The listing builds one solid part. Answer for the finished solid, in the listing's coordinates (mm). A direction names the side the tool comes from. Give positions to 0.01 mm unless a question says otherwise; leave off trailing zeros. Order: outer loops, then holes, each group sorted by start corner. A loop starts at its lowest first (then second) coordinate and runs counter-clockwise, first axis right, second up. Notation, with made-up numbers: (37, 80) - (63, 80) arc R28 cw to (63, 112) - close; hole circle Ø8 at (51, 19.5). An arc over 180 degrees is marked (long way). Use a Markdown table: item, result. Add a question column.
1) The mould has two halves that part along Z. Classify faces 6 (the face through (4.8, 22, -98)), 7 (the face through (4, 33, 0)), 8 (the face through (28.946, 30.8, -86.999)): released by +Z, released by -Z, zero draft, split by the parting line, or undercut.
2) Find section A-A, the plane y = 41. Determine the outline of the cut face in (x, z).
3) Straight lines are drawn through the part: line 1 (X direction, y = 39.5, z = -66.5); line 2 (Y direction, x = 27, z = -159.5); line 3 (Z direction, x = 29, y = 35). For each, find the intervals that lie inside material, in ascending order.
4) Find section C-C, the plane z = -106. Determine the outline of the cut face in (x, y), plus the area to 3 significant figures.
5) For faces 1 (the face through (25.8, 33, -98)), 2 (the face through (4, 33, -199.5)), 3 (the face through (28.946, 30.751, -12.8)), 4 (the face through (28, 23, -98)), 5 (the face through (0, 24, -98)), determine the directions among +Z, -Z, +X, -X, +Y, -Y from which every point of the face is accessible in a straight line to the end or side of a thin tool.
6) Flat-ended cylindrical pins translate along their axes: pin 1 (5 mm diameter, centred on y = 27, z = -78.5, fed in from -X); pin 2 (5.5 mm diameter, centred on x = 28.5, z = -96, fed in from -Y); pin 3 (6 mm diameter, centred on y = 6.5, z = -142.5, fed in from +X). Find the tip coordinate at first contact, or state that the pin passes through.
7) Find section D-D, the plane x = 23.5. Determine the outline of the cut face in (y, z).
8) Find section B-B, the plane z = -167. Determine the outline of the cut face in (x, y), plus the area to 3 significant figures.
from build123d import *

# Parameters (mm, degrees)
BOSS_EXTRUDE1_DEPTH = 199.5
CUT_EXTRUDE1_DEPTH  = 5
CHAMFER1_SIZE       = 3


with BuildPart() as part:
    # Sketch1 → Boss-Extrude1 (new body)
    with BuildSketch(Plane.XY):
        Polygon((0, 0), (0, 49), (30.8, 49), (30.8, 23), (25.8, 23), (25.8, 44), (4.8, 44), (4.8, 0), (7.15, 0), (7.15, -2.7), (-2.35, -2.7), (-2.35, 0), align=None)
    extrude(amount=-BOSS_EXTRUDE1_DEPTH)

    # Sketch2 → Cut-Extrude1 (cut)
    with BuildSketch(Plane(origin=(30.8, 0, 0), x_dir=(0, 0, -1), z_dir=(1, 0, 0))):
        with BuildLine():
            Line((15, 36), (84.75, 36))
            ThreePointArc((84.75, 36), (86.164213562, 35.414213562), (86.75, 34))
            Line((86.75, 34), (86.75, 33))
            ThreePointArc((86.75, 33), (86.164213562, 31.585786438), (84.75, 31))
            Line((84.75, 31), (15, 31))
            ThreePointArc((15, 31), (13.585786438, 31.585786438), (13, 33))
            Line((13, 33), (13, 34))
            ThreePointArc((13, 34), (13.585786438, 35.414213562), (15, 36))
        make_face()
        with BuildLine():
            Line((114.75, 36), (184.5, 36))
            ThreePointArc((184.5, 36), (185.914213562, 35.414213562), (186.5, 34))
            Line((186.5, 34), (186.5, 33))
            ThreePointArc((186.5, 33), (185.914213562, 31.585786438), (184.5, 31))
            Line((184.5, 31), (114.75, 31))
            ThreePointArc((114.75, 31), (113.335786438, 31.585786438), (112.75, 33))
            Line((112.75, 33), (112.75, 34))
            ThreePointArc((112.75, 34), (113.335786438, 35.414213562), (114.75, 36))
        make_face()
    extrude(amount=-CUT_EXTRUDE1_DEPTH, mode=Mode.SUBTRACT)

    # Chamfer1
    chamfer1_edges = [part.edges().sort_by_distance(p)[0] for p in [
        (30.8, 31.585786438, -185.914213562),
        (30.8, 33.5, -186.5),
        (30.8, 35.414213562, -185.914213562),
        (30.8, 36, -149.625),
        (30.8, 35.414213562, -113.335786438),
        (30.8, 33.5, -112.75),
        (30.8, 31.585786438, -113.335786438),
        (30.8, 31, -149.625),
        (30.8, 31.585786438, -86.164213562),
        (30.8, 33.5, -86.75),
        (30.8, 35.414213562, -86.164213562),
        (30.8, 36, -49.875),
        (30.8, 35.414213562, -13.585786438),
        (30.8, 33.5, -13),
        (30.8, 31.585786438, -13.585786438),
        (30.8, 31, -49.875),
    ]]
    chamfer(chamfer1_edges, length=CHAMFER1_SIZE)


solid = part.part
The answers:
| question | item | result |
|---|---|---|
| 1 | face 6 | zero draft |
| 1 | face 7 | released by +Z |
| 1 | face 8 | undercut |
| 2 | outline | (0, -199.5) - (4.8, -199.5) - (4.8, 0) - (0, 0) - close; (25.8, -199.5) - (30.8, -199.5) - (30.8, 0) - (25.8, 0) - close |
| 3 | line 1 | 0 to 4.8, 25.8 to 30.8 |
| 3 | line 2 | 23 to 31, 36 to 49 |
| 3 | line 3 | -199.5 to -187.54, -111.71 to -87.79, -11.96 to 0 |
| 4 | outline | (-2.35, -2.7) - (7.15, -2.7) - (7.15, 0) - (4.8, 0) - (4.8, 44) - (25.8, 44) - (25.8, 23) - (30.8, 23) - (30.8, 49) - (0, 49) - (0, 0) - (-2.35, 0) - close |
| 4 | area | 496 mm2 |
| 5 | face 1 | +Z, -Z, -Y |
| 5 | face 2 | -Z, +X, -X, +Y, -Y |
| 5 | face 3 | +X |
| 5 | face 4 | +Z, -Z, +X, -Y |
| 5 | face 5 | +Z, -Z, -X, +Y |
| 6 | pin 1 | x = 0 |
| 6 | pin 2 | y = 23 |
| 6 | pin 3 | x = 4.8 |
| 7 | outline | (44, -199.5) - (49, -199.5) - (49, 0) - (44, 0) - close |
| 8 | outline | (-2.35, -2.7) - (7.15, -2.7) - (7.15, 0) - (4.8, 0) - (4.8, 44) - (25.8, 44) - (25.8, 36) - (27.8, 36) - (30.8, 39) - (30.8, 49) - (0, 49) - (0, 0) - (-2.35, 0) - close; (25.8, 23) - (30.8, 23) - (30.8, 28) - (27.8, 31) - (25.8, 31) - close |
| 8 | area | 462 mm2 |
